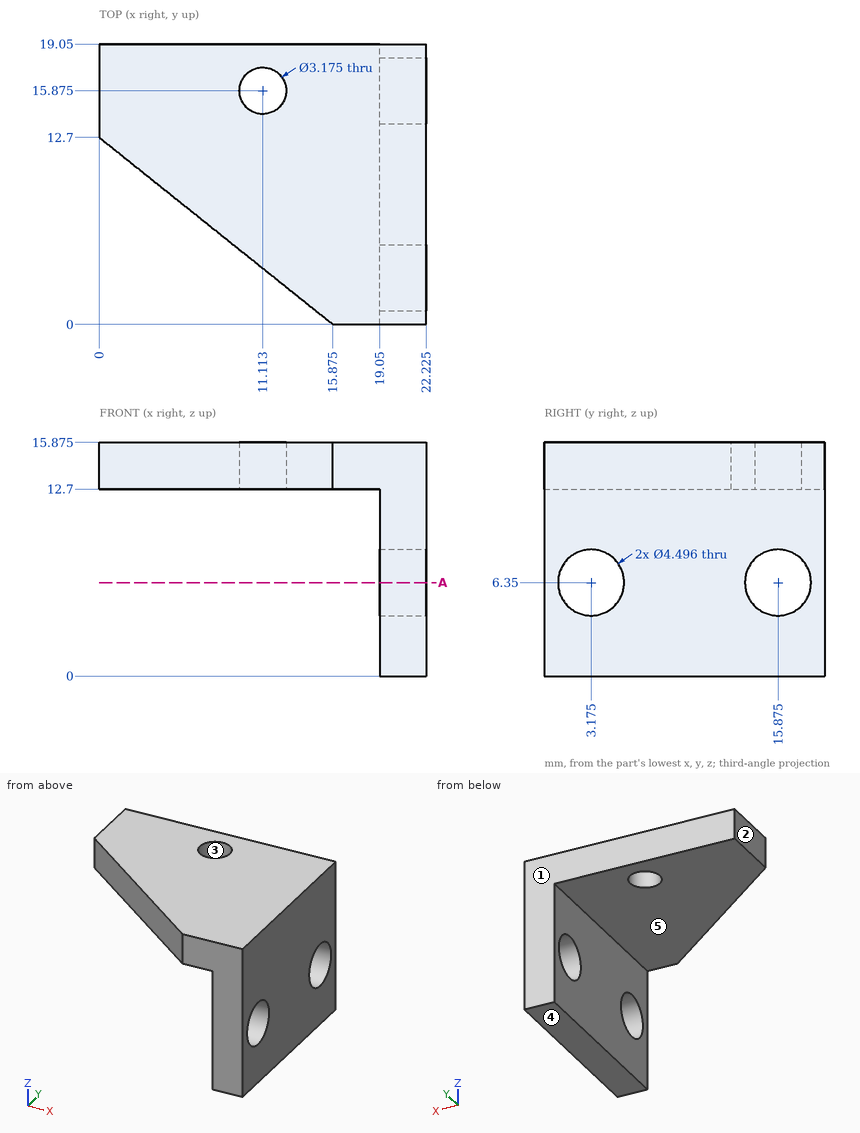
Study the drawing (mm; zero at the part's minimum x, y, z) and answer. A direction names the side the tool comes from. Coordinates: 2 decimals unless noted, no trailing zeros. Write each question's results on one line, items separated by ' | '. Start each with the question number.
1) A tool of negligible diameter and unlimited length cuts with its end or side. For the marked faces 4 and 5, from which of +Z, -Z, +X, -X, +Y, -Y can it reach the whole face along a straight path? Write none if from no direction.
2) For a pull along Y with two mould halves and no side action, classify the marked faces 1, 2 and 3 as +Y half, -Y half, draft (parallel to the pull), parting line (faces both ways), or undercut.
3) Straight lines are drawn through the part: probe 1 along Y at (x, z) = (20.4, 6.35); probe 2 along Z at (x, y) = (7, 9) (1 decimal); probe 3 along Z at (x, y) = (20, 1.25) (1 decimal). For each, find the intervals that lie inside material, in ascending order.
4) A cutting plane is placed at A-A (z = 6.35). Count the separate pieces of the cut face and the enclosed holes in it.
5) Flat-ended cylindrical pins translate along their axes: pin 1 Ø3 at (x, z) = (15.5, 11) entering from -Y; pin 2 Ø3 at (y, z) = (13.5, 4.5) entering from -X; pin 3 Ø5 at (y, z) = (10, 11) entering from -X (1 decimal). Find the tip coordinate at first contact, or state that the pin passes through.
Values follow:
1) face 4: -Z, +X, -X, +Y, -Y | face 5: -Z, -X, +Y, -Y
2) face 1: +Y half | face 2: draft | face 3: undercut
3) probe 1: 0 to 0.93, 5.42 to 13.63, 18.12 to 19.05 | probe 2: 12.7 to 15.9 | probe 3: 0 to 5.2, 7.5 to 15.9
4) separate pieces: 3 | enclosed holes: 0
5) pin 1: through | pin 2: x = 19.05 | pin 3: x = 1.1
